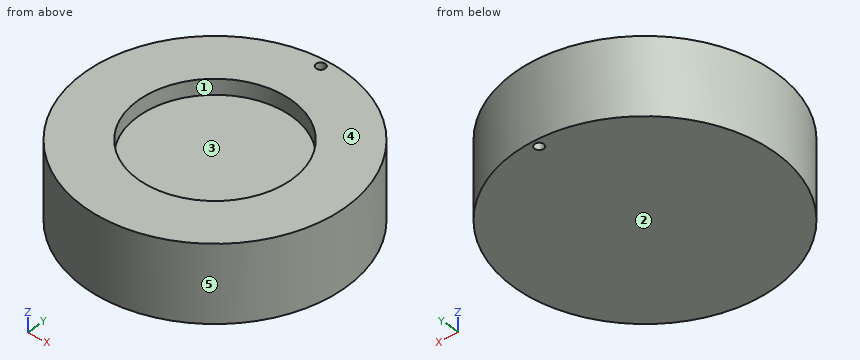
```python
from build123d import *

# Parameters (mm, degrees)
F0_R     = 42.5
F0_R_2   = 25
F0_R_3   = 1.5
F1_DEPTH = 5
F2_DEPTH = 20
F3_DEPTH = 25


with BuildPart() as f1:
    # F0 (on Top) → F1 (new body)
    with BuildSketch(Plane.XY):
        Circle(F0_R)
        Circle(F0_R_2, mode=Mode.SUBTRACT)
        with Locations((0, 39.939713)):
            Circle(F0_R_3, mode=Mode.SUBTRACT)
        Circle(F0_R_2)
    extrude(amount=F1_DEPTH)

    # F0 (on Top) → F2 (join)
    with BuildSketch(Plane.XY):
        Circle(F0_R_2)
    extrude(amount=F2_DEPTH)

    # F0 (on Top) → F3 (join)
    with BuildSketch(Plane.XY):
        Circle(F0_R)
        Circle(F0_R_2, mode=Mode.SUBTRACT)
        with Locations((0, 39.939713)):
            Circle(F0_R_3, mode=Mode.SUBTRACT)
    extrude(amount=F3_DEPTH)


solid = f1.part
```
Geometry check sheet. Reference: the model listing, model coordinates, mm. Face numbers are marked on the shaded views. A direction names the side the tool comes from. Give positions to 0.01 mm unless a question says otherwise; leave off trailing zeros. Write each loop counter-clockwise with the first axis right and the second up, starting at its lowest first coordinate (ties: lowest second). Pieces come first, ordered by that corner, then holes.
1) Section check B-B, the plane y = -12. Record the boundary of the cut face in (x, z), and give its area (3 significant figures).
2) Material ranges on L1, parallel to Y at x = 0, z = 22.2; L2, parallel to Y at x = 0, z = 6.5; L3, parallel to Z at x = -10.5, y = 0, recorded low to high.
3) Section check C-C, the plane x = 23.5. Record the boundary of the cut face in (y, z), and give its area (3 significant figures).
4) Section check D-D, the plane z = 11. Record the boundary of the cut face in (x, y).
5) Gauge pin test, flat ends, axial feed: pin 1 (5 mm diameter, centred on x = 34, z = 9.5, fed in from +Y); pin 2 (10 mm diameter, centred on y = -20.5, z = 21.5, fed in from -X); pin 3 (1.5 mm diameter, centred on y = -15, z = 9, fed in from +X). Record the tip position at first contact, or that the pin passes through.
6) Release check for a two-part mould opening along X. For the marked faces 3, 4 and 5 record: pulls with the +X half, pulls with the -X half, needs draft (parallel to the pull), parting line crosses it, or undercut.
7) Access from +Z, -Z, +X, -X, +Y, -Y to the whole of each face (thin tool, end or side, straight path). Record for the marked faces 1 and 2.
8) Section check A-A, the plane x = 0. Record the boundary of the cut face in (y, z).
Computed:
1. outline: (-40.77, 0) - (40.77, 0) - (40.77, 25) - (21.93, 25) - (21.93, 20) - (-21.93, 20) - (-21.93, 25) - (-40.77, 25) - close
1. area: 1,820 mm2
2. L1: y = -42.5 to -25, 25 to 38.44, 41.44 to 42.5
2. L2: y = -42.5 to 38.44, 41.44 to 42.5
2. L3: z = 0 to 20
3. outline: (-35.41, 0) - (35.41, 0) - (35.41, 25) - (8.53, 25) - (8.53, 20) - (-8.53, 20) - (-8.53, 25) - (-35.41, 25) - close
3. area: 1,690 mm2
4. outline: circle Ø85 at (0, 0); hole circle Ø3 at (0, 39.94)
5. pin 1: stops at y = 28.53
5. pin 2: stops at x = -39.57
5. pin 3: stops at x = 40.04
6. face 3: undercut
6. face 4: needs draft
6. face 5: parting line crosses it
7. face 1: +Z
7. face 2: -Z, +X, -X, +Y, -Y
8. outline: (-42.5, 0) - (38.44, 0) - (38.44, 25) - (25, 25) - (25, 20) - (-25, 20) - (-25, 25) - (-42.5, 25) - close; (41.44, 0) - (42.5, 0) - (42.5, 25) - (41.44, 25) - close
